Input: part model. Units: mm. Frame: model coordinates. Round coordinates to 2 decimals unless told otherwise and drop trailing zeros. Loops run counter-clockwise (first coordinate to the right, second up) from the corner with the lowest first, then second, coordinate; pieces in that order, holes last. Notation, with made-up numbers: (-31, 10.25) -> (-8, 10.25) arc R16 cw to (-8, 30.25) -> close; hole circle Ø4 at (-35.5, -29). An arc over 180 degrees is marked (long way). One line per question, with ' | ' between items. Start each with the question number.
Q1. Material intervals for L1, parallel to X at y = 2.1, z = -278; L2, parallel to X at y = 2.55, z = 49; L3, parallel to X at y = 0.35, z = -45.5, sorted ascending.
Q2. Cut plane B-B on z = 138. Return loops of the section in (x, y).
Q3. Cut plane A-A on x = -10. Return loops of the section in (y, z), and give its area (3 significant figures).
Q4. Contact query for flat-ended pins moving along their axis: P1, Ø3, axis at x = 157, y = 1, coming from the +Z side; P2, Ø3.5, axis at x = -46.48, z = -278, coming from the +Y side; P3, Ø2, axis at y = 1, z = -135.5, coming from the -X side. Output: stop coordinate, or through.
Q5. Cut plane D-D on y = 3.15. State how many separate pieces and enclosed holes the cut face has, and give its area (3 significant figures).
Q6. Mould query, pull axis X, two halves, no side actions, for faces 1 (the face through (-6, 0, 62)), 2 (the face through (-182, 3, 168)), 3 (the face through (-31.065, 2.958, -50.806)). Classes: pulls with the +X half, pulls with the -X half, needs draft (parallel to the pull), parting line crosses it, or undercut.
Q7. Cut plane C-C on x = 179. Return loops of the section in (y, z).
from build123d import *

# Parameters (mm, degrees)
BOSS_EXTRUDE1_DEPTH       = 6
SKETCH4_R                 = 0.495653738
CUT_EXTRUDE3_DEPTH        = 10
BOSS_EXTRUDE3_DEPTH       = 6
SKETCH6_R                 = 2
SKETCH6_R_2               = 4
CUT_EXTRUDE4_DEPTH        = 12
CIRPATTERN1_COUNT         = 4
BOSS_EXTRUDE4_DEPTH       = 6
F_4_0MM_DOWEL_HOLE5_D     = 4
F_4_0MM_DOWEL_HOLE5_DEPTH = 25.4
F_4_0MM_DOWEL_HOLE5_TIP   = 1.201721238
F_4_0MM_DOWEL_HOLE4_D     = 4
F_4_0MM_DOWEL_HOLE4_DEPTH = 98.31
F_4_0MM_DOWEL_HOLE4_TIP   = 1.201721238
SKETCH31_R                = 55
CUT_EXTRUDE7_DEPTH        = 22
SKETCH32_R                = 3.837227577
SKETCH32_R_2              = 3.691246821
SKETCH32_R_3              = 4.005777273
SKETCH32_R_4              = 3.413782358
SKETCH32_R_5              = 2.946286388
SKETCH32_R_6              = 2.662859758
SKETCH32_R_7              = 3.21029216
SKETCH32_R_8              = 3.304223232
SKETCH32_R_9              = 3.416276983
SKETCH32_R_10             = 5.576814982
SKETCH32_R_11             = 3.327214885
SKETCH32_R_12             = 3.217650006
SKETCH32_R_13             = 3.084152149
SKETCH32_R_14             = 2.850354754
SKETCH32_R_15             = 3.581653386
SKETCH32_R_16             = 3.209735743
SKETCH32_R_17             = 5.223630371
SKETCH32_R_18             = 3.239996293
SKETCH32_R_19             = 6.217574628
SKETCH32_R_20             = 3.281482388
SKETCH32_R_21             = 4.010466873
SKETCH32_R_22             = 4.080831309
SKETCH32_R_23             = 4.290737966
SKETCH32_R_24             = 4.085305416
SKETCH32_R_25             = 4.488085615
SKETCH32_R_26             = 4.89911642
SKETCH32_R_27             = 5.474778022
SKETCH32_R_28             = 7.813771611
SKETCH32_R_29             = 3.187569437
SKETCH32_R_30             = 2.929784552
SKETCH32_R_31             = 4.009606332
SKETCH32_R_32             = 4.090801563
BOSS_EXTRUDE5_DEPTH       = 6


with BuildPart() as part:
    # Sketch1 → Boss-Extrude1 (new body)
    with BuildSketch(Plane(origin=(0, 0, 0), x_dir=(1, 0, 0), z_dir=(0, 1, 0))):
        with BuildLine():
            Line((-110, 50), (-300, 50))
            ThreePointArc((-300, 50), (-307.071067812, 47.071067812), (-310, 40))
            Line((-310, 40), (-310, -40))
            ThreePointArc((-310, -40), (-307.071067812, -47.071067812), (-300, -50))
            Line((-300, -50), (-110, -50))
            Line((-110, -50), (-60, -100))
            Line((-60, -100), (-60, -290))
            ThreePointArc((-60, -290), (-57.071067812, -297.071067812), (-50, -300))
            Line((-50, -300), (30, -300))
            ThreePointArc((30, -300), (37.071067812, -297.071067812), (40, -290))
            Line((40, -290), (40, -100))
            Line((40, -100), (90, -50))
            Line((90, -50), (280, -50))
            ThreePointArc((280, -50), (287.071067812, -47.071067812), (290, -40))
            Line((290, -40), (290, 40))
            ThreePointArc((290, 40), (287.071067812, 47.071067812), (280, 50))
            Line((280, 50), (90, 50))
            Line((90, 50), (40, 100))
            Line((40, 100), (40, 290))
            ThreePointArc((40, 290), (37.071067812, 297.071067812), (30, 300))
            Line((30, 300), (-50, 300))
            ThreePointArc((-50, 300), (-57.071067812, 297.071067812), (-60, 290))
            Line((-60, 290), (-60, 100))
            Line((-60, 100), (-110, 50))
        make_face()
    extrude(amount=BOSS_EXTRUDE1_DEPTH)

    # Sketch4 → Cut-Extrude3 (cut)
    with BuildSketch(Plane(origin=(0, 6, 0), x_dir=(1, 0, 0), z_dir=(0, 1, 0))):
        with Locations(Location((-10, 0, 0), (0, 0, 270))):
            Circle(SKETCH4_R)
    extrude(amount=-CUT_EXTRUDE3_DEPTH, mode=Mode.SUBTRACT)

    # Sketch5 → Boss-Extrude3 (add)
    with BuildSketch(Plane(origin=(0, 6, 0), x_dir=(1, 0, 0), z_dir=(0, 1, 0))):
        Polygon((-300, 50), (-60, 290), (-60, 240), (-250, 50), align=None)
        Polygon((40, 290), (280, 50), (230, 50), (40, 240), align=None)
        Polygon((280, -50), (40, -290), (40, -240), (230, -49.07797178), align=None)
        Polygon((-300, -50), (-60, -290), (-60, -240), (-250, -50), align=None)
    extrude(amount=-BOSS_EXTRUDE3_DEPTH)

    # Sketch6 → Cut-Extrude4 (cut)
    with BuildSketch(Plane(origin=(0, 6, 0), x_dir=(1, 0, 0), z_dir=(0, 1, 0))):
        with Locations(Location((-37.824146891, 287.83697558, 0), (0, 0, 270))):
            Circle(SKETCH6_R)
        with Locations(Location((-37.824146891, 272.83697558, 0), (0, 0, 270))):
            Circle(SKETCH6_R)
        with Locations(Location((-46.483109463, 221.536893944, 0), (0, 0, 270))):
            Circle(SKETCH6_R)
        with Locations(Location((-46.483109463, 135.06793836, 0), (0, 0, 270))):
            Circle(SKETCH6_R)
        with Locations(Location((-69.817594081, 73.334484618, 0), (0, 0, 270))):
            Circle(SKETCH6_R)
        with Locations(Location((49.817594081, 73.334484618, 0), (0, 0, 270))):
            Circle(SKETCH6_R)
        with Locations(Location((26.483109463, 135.06793836, 0), (0, 0, 270))):
            Circle(SKETCH6_R)
        with Locations(Location((26.483109463, 221.536893944, 0), (0, 0, 270))):
            Circle(SKETCH6_R)
        with Locations(Location((191.360389693, 113.639610307, 0), (0, 0, 270))):
            Circle(SKETCH6_R)
        with Locations(Location((128.639610307, 176.360389693, 0), (0, 0, 270))):
            Circle(SKETCH6_R)
        with Locations(Location((17.824146891, 272.83697558, 0), (0, 0, 270))):
            Circle(SKETCH6_R)
        with Locations(Location((17.824146891, 287.83697558, 0), (0, 0, 270))):
            Circle(SKETCH6_R)
        with Locations(Location((-10, 0, 0), (0, 0, 270))):
            Circle(SKETCH6_R_2)
    cut_extrude4 = extrude(amount=-CUT_EXTRUDE4_DEPTH, mode=Mode.SUBTRACT)

    # CirPattern1: Cut-Extrude4 ×4 about axis
    cirpattern1_axis = Axis((-10, 0, 0), (0, 1, 0))
    for i in range(1, CIRPATTERN1_COUNT):
        add(cut_extrude4.rotate(cirpattern1_axis, i * 360 / CIRPATTERN1_COUNT), mode=Mode.SUBTRACT)

    # Sketch7 → Boss-Extrude4 (add)
    with BuildSketch(Plane(origin=(0, 6, 0), x_dir=(1, 0, 0), z_dir=(0, 1, 0))):
        Polygon((40, 240), (230, 50), (90, 50), (40, 100), align=None)
        Polygon((90, -50), (229.082424571, -50), (40, -240), (40, -100), align=None)
        Polygon((-60, 240), (-60, 100), (-110, 50), (-250, 50), align=None)
        Polygon((-110, -50), (-60, -100), (-60, -240), (-250, -50), align=None)
    extrude(amount=-BOSS_EXTRUDE4_DEPTH)

    # Ø4.0mm Dowel Hole5
    with Locations(Plane(origin=(0, 6, 0), x_dir=(1, 0, 0), z_dir=(0, 1, 0))):
        with Locations((-29.100763253, 23.781275186), (32.712886556, 23.781275186), (31.383087371, -32.5), (-30.430562437, -32.5)):
            Hole(F_4_0MM_DOWEL_HOLE5_D / 2, depth=F_4_0MM_DOWEL_HOLE5_DEPTH)
            with Locations((0, 0, -(F_4_0MM_DOWEL_HOLE5_DEPTH + F_4_0MM_DOWEL_HOLE5_TIP / 2))):  # 118° drill point
                Cone(0, F_4_0MM_DOWEL_HOLE5_D / 2, F_4_0MM_DOWEL_HOLE5_TIP, mode=Mode.SUBTRACT)

    # Ø4.0mm Dowel Hole4
    with Locations(Plane(origin=(0, 0, 0), x_dir=(-1, 0, 0), z_dir=(0, -1, 0))):
        with Locations((46.483109463, -278), (-26.483109463, -278), (-268, -36.483109463), (-268, 36.483109463), (-26.483109463, 278), (46.483109463, 278), (288, 36.483109463), (288, -36.483109463)):
            Hole(F_4_0MM_DOWEL_HOLE4_D / 2, depth=F_4_0MM_DOWEL_HOLE4_DEPTH)
            with Locations((0, 0, -(F_4_0MM_DOWEL_HOLE4_DEPTH + F_4_0MM_DOWEL_HOLE4_TIP / 2))):  # 118° drill point
                Cone(0, F_4_0MM_DOWEL_HOLE4_D / 2, F_4_0MM_DOWEL_HOLE4_TIP, mode=Mode.SUBTRACT)

    # Sketch31 → Cut-Extrude7 (cut)
    with BuildSketch(Plane.XZ):
        with Locations(Location((-10, 0, 0), (0, 0, 270))):
            Circle(SKETCH31_R)
    extrude(amount=-CUT_EXTRUDE7_DEPTH, mode=Mode.SUBTRACT)

    # Sketch32 → Boss-Extrude5 (add)
    with BuildSketch(Plane.XZ):
        with Locations((-148.639610307, 176.360389693)):
            Circle(SKETCH32_R)
        with Locations((-211.360389693, 113.639610307)):
            Circle(SKETCH32_R_2)
        with Locations((-282.83697558, 27.824146891)):
            Circle(SKETCH32_R_3)
        with Locations((-297.83697558, 27.824146891)):
            Circle(SKETCH32_R_4)
        with Locations((-297.83697558, -27.824146891)):
            Circle(SKETCH32_R_5)
        with Locations((-282.83697558, -27.824146891)):
            Circle(SKETCH32_R_6)
        with Locations((-145.06793836, -36.483109463)):
            Circle(SKETCH32_R_7)
        with Locations((-145.06793836, 36.457377156)):
            Circle(SKETCH32_R_8)
        with Locations((-186.360389693, -138.639610307)):
            Circle(SKETCH32_R_9)
        with Locations((-123.838638112, -202.788762732)):
            Circle(SKETCH32_R_10)
        with Locations((-37.824146891, -272.83697558)):
            Circle(SKETCH32_R_11)
        with Locations((-37.824146891, -287.83697558)):
            Circle(SKETCH32_R_12)
        with Locations((17.824146891, -287.83697558)):
            Circle(SKETCH32_R_13)
        with Locations((17.824146891, -272.83697558)):
            Circle(SKETCH32_R_14)
        with Locations((26.483109463, -135.06793836)):
            Circle(SKETCH32_R_15)
        with Locations((-46.483109463, -135.06793836)):
            Circle(SKETCH32_R_16)
        with Locations((128.639610307, -176.360389693)):
            Circle(SKETCH32_R_17)
        with Locations((125.06793836, -37.248921052)):
            Circle(SKETCH32_R_18)
        with Locations((190.399105171, -114.010951532)):
            Circle(SKETCH32_R_19)
        with Locations((125.253969426, 35.650797055)):
            Circle(SKETCH32_R_20)
        with Locations((277.982195025, 26.611427969)):
            Circle(SKETCH32_R_21)
        with Locations((262.862191843, 26.611427969)):
            Circle(SKETCH32_R_22)
        with Locations((261.817821155, -27.824146891)):
            Circle(SKETCH32_R_23)
        with Locations((277.008476777, -28.651243723)):
            Circle(SKETCH32_R_24)
        with Locations((25.470022372, 134.658293559)):
            Circle(SKETCH32_R_25)
        with Locations((-46.142219861, 134.074156368)):
            Circle(SKETCH32_R_26)
        with Locations((102.990893209, 200.50311812)):
            Circle(SKETCH32_R_27)
        with Locations((165.946806213, 137.06793836)):
            Circle(SKETCH32_R_28)
        with Locations((17.414125568, 272.231636603)):
            Circle(SKETCH32_R_29)
        with Locations((17.181225285, 287.538992514)):
            Circle(SKETCH32_R_30)
        with Locations((-38.293050813, 286.797735955)):
            Circle(SKETCH32_R_31)
        with Locations((-38.831274267, 271.695880736)):
            Circle(SKETCH32_R_32)
    extrude(amount=-BOSS_EXTRUDE5_DEPTH)


solid = part.part
Results:
1) L1: -72 to -48.48, -44.48 to 24.48, 28.48 to 52 | L2: -304.36 to -34.98, 14.98 to 284.36 | L3: -308.35 to -40.9, 20.9 to 288.35
2) outline: (-212, 0) -> (192, 0) -> (192, 6) -> (-212, 6) -> close
3) outline: (0, -300) -> (6, -300) -> (6, -55) -> (0, -55) -> close; (0, 55) -> (6, 55) -> (6, 300) -> (0, 300) -> close | area: 2,940 mm^2
4) P1: z = 174.5 | P2: through | P3: x = -215.5
5) separate pieces: 1 | enclosed holes: 25 | area: 215,000 mm^2
6) face 1: needs draft | face 2: pulls with the -X half | face 3: undercut
7) outline: (0, -151) -> (6, -151) -> (6, 151) -> (0, 151) -> close
